from build123d import *

# Parameters (mm, degrees)
SKIZZE1_W                                           = 100
SKIZZE1_H                                           = 50
AUFSATZ_LINEAR_AUSTRAGEN1_DEPTH                     = 100
STIRNSENKUNG_F_R_M8_SENKSCHRAUBE_KOPF_B_D           = 9
STIRNSENKUNG_F_R_M8_SENKSCHRAUBE_KOPF_B_CBORE_D     = 15
STIRNSENKUNG_F_R_M8_SENKSCHRAUBE_KOPF_B_CBORE_DEPTH = 45
STIRNSENKUNG_F_R_M8_SENKSCHRAUBE_KO_2_D             = 9
STIRNSENKUNG_F_R_M8_SENKSCHRAUBE_KO_2_CBORE_D       = 15
STIRNSENKUNG_F_R_M8_SENKSCHRAUBE_KO_2_CBORE_DEPTH   = 116


# Read off the part's stored shape, not the designer's step: Kernloch für M8 Helicoil1
with BuildPart() as part:
    # Skizze1 → Aufsatz-Linear austragen1 (new body)
    with BuildSketch(Plane.XY):
        Rectangle(SKIZZE1_W, SKIZZE1_H)
    extrude(amount=AUFSATZ_LINEAR_AUSTRAGEN1_DEPTH)

    # Stirnsenkung f_r M8 Senkschraube _Kopf B (through all)
    with Locations(Plane(origin=(0, 25, 0), x_dir=(1, 0, 0), z_dir=(0, 1, 0))):
        with Locations((35, -85), (-35, -15)):
            CounterBoreHole(STIRNSENKUNG_F_R_M8_SENKSCHRAUBE_KOPF_B_D / 2, STIRNSENKUNG_F_R_M8_SENKSCHRAUBE_KOPF_B_CBORE_D / 2, STIRNSENKUNG_F_R_M8_SENKSCHRAUBE_KOPF_B_CBORE_DEPTH)

    # Stirnsenkung f_r M8 Senkschraube _Ko 2 (through all)
    with Locations(Plane.XY.offset(100)):
        with Locations((0, 0)):
            CounterBoreHole(STIRNSENKUNG_F_R_M8_SENKSCHRAUBE_KO_2_D / 2, STIRNSENKUNG_F_R_M8_SENKSCHRAUBE_KO_2_CBORE_D / 2, STIRNSENKUNG_F_R_M8_SENKSCHRAUBE_KO_2_CBORE_DEPTH)

    # Kernloch für M8 Helicoil1 outline → Kernloch für M8 Helicoil1 (revolve, cut)
    with BuildSketch(Plane(origin=(17.5, 0, 35), x_dir=(1, 0, 0), z_dir=(0, 0, 1))):
        Polygon((0, 25), (0, 2.506428431), (4.15, 5), (4.15, 25), align=None)
    revolve(axis=Axis((17.5, 0, 35), (0, 1, 0)), mode=Mode.SUBTRACT)

    # Kernloch f_r M8 Helicoil1 2 outline → Kernloch f_r M8 Helicoil1 2 (revolve, cut)
    with BuildSketch(Plane(origin=(-17.5, 0, 35), x_dir=(1, 0, 0), z_dir=(0, 0, 1))):
        Polygon((0, 25), (0, 2.506428431), (4.15, 5), (4.15, 25), align=None)
    revolve(axis=Axis((-17.5, 0, 35), (0, 1, 0)), mode=Mode.SUBTRACT)


solid = part.part
Work out the finished part from the listing and answer in its coordinate system (mm). A direction names the side the tool comes from. Coordinates: 2 decimals unless noted, no trailing zeros. Loops run counter-clockwise (first coordinate to the right, second up) from the corner with the lowest first, then second, coordinate; pieces in that order, holes last. Notation, with made-up numbers: M 30,-22 L 74,-22 A17 ccw 74,-15 Z; hole C 79.25,80 d2. An arc over 180 degrees is marked long. Answer in a Markdown table with one row per item. Add a question column.
1. Consider L1, parallel to Z at x = -35, y = 8; L2, parallel to Z at x = -17, y = 16; L3, parallel to X at y = 4, z = 80.5. Determine where each line is inside the solid, lowest interval first.
2. Flat-ended cylindrical pins translate along their axes: P1, Ø9, axis at x = 0, y = 0, coming from the -Z side; P2, Ø13.5, axis at x = -35, z = 15, coming from the +Y side; P3, Ø5, axis at x = -17.5, z = 35, coming from the +Y side. Find the tip coordinate at first contact, or state that the pin passes through.
3. Find section C-C, the plane x = -35. Write down the section's boundary in (y, z), then the cut area to 3 significant figures.
4. Find section D-D, the plane y = 10.5. Write down the section's boundary in (x, z).
5. Find section A-A, the plane y = 0. Write down the section's boundary in (x, z).
6. A tool of negligible diameter and unlimited length cuts with its end or side. For faces 5 (the cylindrical face through (-39.292, -22.535, 13.648)), 6 (the cylindrical face through (-42.493, 2.815, 14.67)), from which of +Z, -Z, +X, -X, +Y, -Y can it reach the whole face along a straight path? Write none if from no direction.
7. The mould has two halves that part along Z. Classify faces 1 (the flat face through (50, 0, 49)), 2 (the cylindrical face through (14.441, 15.14, 32.195)), 3 (the conical face through (16.97, 2.94, 34.51)), 4 (the flat face through (-1, 11, 0)): pulls with the +Z half, pulls with the -Z half, needs draft (parallel to the pull), parting line crosses it, or undercut.
8. Find section B-B, the plane z = 15. Write down the section's boundary in (x, y), then the cut area to 3 significant figures.
Reported:
| question | item | result |
|---|---|---|
| 1 | L1 | z = 0 to 7.5, 22.5 to 100 |
| 1 | L2 | z = 0 to 30.88, 39.12 to 100 |
| 1 | L3 | x = -50 to -6.34, 6.34 to 29, 41 to 50 |
| 2 | P1 | passes through |
| 2 | P2 | stops at y = -20 |
| 2 | P3 | stops at y = 4.01 |
| 3 | outline | M -25,0 L 25,0 L 25,7.5 L -20,7.5 L -20,10.5 L -25,10.5 Z; M -25,19.5 L -20,19.5 L -20,22.5 L 25,22.5 L 25,100 L -25,100 Z |
| 3 | area | 4,280 mm^2 |
| 4 | outline | M -50,0 L 50,0 L 50,100 L -50,100 Z; hole C -35,15 d15; hole C -17.5,35 d8.3; hole C 17.5,35 d8.3; hole C 35,85 d15 |
| 5 | outline | M -50,0 L -7.5,0 L -7.5,100 L -50,100 Z; M 7.5,0 L 50,0 L 50,100 L 7.5,100 Z; hole C -35,15 d15; hole C 35,85 d15 |
| 6 | face 5 | +Y, -Y |
| 6 | face 6 | +Y |
| 7 | face 1 | needs draft |
| 7 | face 2 | undercut |
| 7 | face 3 | undercut |
| 7 | face 4 | pulls with the -Z half |
| 8 | outline | M -50,-25 L -39.5,-25 L -39.5,-20 L -42.5,-20 L -42.5,25 L -50,25 Z; M -30.5,-25 L 50,-25 L 50,25 L -27.5,25 L -27.5,-20 L -30.5,-20 Z; hole C 0,0 d15 |
| 8 | area | 4,100 mm^2 |
